Verification items for the finished model (mm, model axes). A direction names the side the tool comes from. Round coordinates to 2 decimals unless told otherwise and drop trailing zeros. One line per item, written item: value. Start each with the question number.
Item 1: Tool access check on faces 5 (the face through (28.554, -6.341, 19.25)), 6 (the face through (-14.78, 46.94, 52.24)), 7 (the face through (-24.4, 8.5, 421.513)), 8 (the face through (21.784, -28.41, 421.191)). Record the directions out of +Z, -Z, +X, -X, +Y, -Y that give a thin tool (end or side, any length) a straight path to the whole face; none if there is none.
Item 2: Thickness scan on probe 1 along X at (y, z) = (0, -342.5); probe 2 along Y at (x, z) = (0, 416.5); probe 3 along Y at (x, z) = (0, 119). Record the ranges inside material, lowest first. Write a range as from..to.
Item 3: Gauge pin test, flat ends, axial feed: pin 1 (8 mm diameter, centred on y = -5.5, z = -49.5, fed in from +X); pin 2 (4 mm diameter, centred on x = -29, y = -30.5, fed in from -Z); pin 3 (1 mm diameter, centred on y = -33.5, z = 160, fed in from -X). Record the tip position at first contact, or that the pin passes through.
Item 4: Draft check along Y on faces 1 (the face through (-4.372, 13.883, 335.202)), 2 (the face through (21, -12, -293.878)), 3 (the face through (-11.69, 7.46, 342.45)), 4 (the face through (-3.755, 11.923, -337.567)). Enter one of: +Y half, -Y half, draft (parallel to the pull), parting line (faces both ways), or undercut.
from build123d import *

# Parameters (mm, degrees)
CHAMFER1_SIZE                     = 1.5
F_3_8_16_TAPPED_HOLE1_D           = 7.9375
F_3_8_16_TAPPED_HOLE1_DEPTH       = 25.4
F_3_8_16_TAPPED_HOLE1_CSINK_D     = 10.795
F_3_8_16_TAPPED_HOLE1_CSINK_ANGLE = 100
F_3_8_16_TAPPED_HOLE1_TIP         = 2.384665582


with BuildPart() as part:
    # Sketch1 → Revolve1 (revolve)
    with BuildSketch(Plane(origin=(0, 0, 0), x_dir=(0, 0, -1), z_dir=(1, 0, 0))):
        Polygon((-420.878, 50.8), (-408.178, 50.8), (-408.178, 49.2125), (293.878, 49.2125), (293.878, 23.876), (323.723, 23.876), (323.723, 12.5), (351.028, 12.5), (351.028, 0), (271.028, 0), (271.028, 29.25), (-301.513, 29.25), (-301.513, 40.25), (-309.506817629, 40.25), (-336.513, 13.243817629), (-351.513, 14.820381157), (-411.513, 25.4), (-421.513, 25.4), (-421.513, 35.8), (-420.878, 35.8), align=None)
    revolve(axis=Axis((0, 0, -473.12001368), (0, 0, 1)))

    # Chamfer1
    chamfer1_edges = [part.edges().sort_by_distance(p)[0] for p in [
        (0, -23.876, -323.723),
    ]]
    chamfer(chamfer1_edges, length=CHAMFER1_SIZE)

    # 3/8-16 Tapped Hole1
    with Locations(Plane(origin=(0, 0, -351.028), x_dir=(-1, 0, 0), z_dir=(0, 0, -1))):
        with Locations((0, 0)):
            CounterSinkHole(F_3_8_16_TAPPED_HOLE1_D / 2, F_3_8_16_TAPPED_HOLE1_CSINK_D / 2, depth=F_3_8_16_TAPPED_HOLE1_DEPTH, counter_sink_angle=F_3_8_16_TAPPED_HOLE1_CSINK_ANGLE)
            with Locations((0, 0, -(F_3_8_16_TAPPED_HOLE1_DEPTH + F_3_8_16_TAPPED_HOLE1_TIP / 2))):  # 118° drill point
                Cone(0, F_3_8_16_TAPPED_HOLE1_D / 2, F_3_8_16_TAPPED_HOLE1_TIP, mode=Mode.SUBTRACT)


solid = part.part
Response values:
1. face 5: none
1. face 6: -Z
1. face 7: +Z, +X, -X, +Y, -Y
1. face 8: +Z
2. probe 1: x = -12.5..-3.97, 3.97..12.5
2. probe 2: y = -50.8..-25.4, 25.4..50.8
2. probe 3: y = -49.21..-29.25, 29.25..49.21
3. pin 1: stops at x = 49.19
3. pin 2: stops at z = -293.88
3. pin 3: stops at x = -36.51
4. face 1: undercut
4. face 2: draft
4. face 3: undercut
4. face 4: parting line
